Read the model definition and answer for the solid it produces. Units are mm, in the model's axes. A direction names the side the tool comes from. Round coordinates to 2 decimals unless told otherwise and drop trailing zeros. Loops run counter-clockwise (first coordinate to the right, second up) from the corner with the lowest first, then second, coordinate; pieces in that order, holes last. Notation, with made-up numbers: (72.5, 43.25) - (83.5, 43.25) arc R14 ccw to (83.5, 61.25) - close; hole circle Ø7 at (86.5, 56). An arc over 180 degrees is marked (long way). Answer as CSV lines item,"result".
```python
from build123d import *

# Parameters (mm, degrees)
BOSS_EXTRUDE1_DEPTH = 42
CUT_EXTRUDE1_REACH  = 70.337
SKETCH2_W           = 19
SKETCH2_H           = 33
SKETCH3_R           = 2.25
BOSS_EXTRUDE2_DEPTH = 8.75
FILLET1_R           = 0.5


with BuildPart() as part:
    # Sketch1 → Boss-Extrude1 (new body)
    with BuildSketch(Plane.XY):
        Polygon((19.580645161, 0), (19.580645161, 6.5), (4.580645161, 6.5), (4.580645161, 0), (-8.419354839, 0), (-8.419354839, 3), (-8.419354839, 35), (1.580645161, 35), (22.580645161, 35), (22.580645161, 3), (32.580645161, 3), (32.580645161, 0), align=None)
    extrude(amount=BOSS_EXTRUDE1_DEPTH)

    # Cut-Extrude1: up to this face of the body (flat: up to its plane)
    cut_extrude1_end = Plane(part.part.faces().sort_by_distance((4.580645161, 3.25, 21))[0])
    # Sketch2 → Cut-Extrude1 (cut, up to the picked face)
    with BuildSketch(Plane(origin=(32.580645161, 0, 0), x_dir=(0, 0, -1), z_dir=(1, 0, 0)), mode=Mode.PRIVATE) as cut_extrude1_sk1:
        with Locations((-21, 16.5)):
            Rectangle(SKETCH2_W, SKETCH2_H)
    cut_extrude1_tool1 = split(extrude(cut_extrude1_sk1.sketch, amount=-CUT_EXTRUDE1_REACH, mode=Mode.PRIVATE), bisect_by=cut_extrude1_end, keep=Keep.BOTH, mode=Mode.PRIVATE)
    add(cut_extrude1_tool1.solids().sort_by(Axis((32.580645, 16.5, 21), (-1, 0, 0)))[0], mode=Mode.SUBTRACT)

    # Sketch3 → Boss-Extrude2 (add)
    with BuildSketch(Plane(origin=(0, 35, 0), x_dir=(1, 0, 0), z_dir=(0, 1, 0))):
        with Locations(Location((-2.051707365, -21, 0), (0, 0, 90))):
            Circle(SKETCH3_R)
    extrude(amount=BOSS_EXTRUDE2_DEPTH)

    # Fillet1
    fillet1_edges = [part.edges().sort_by_distance(p)[0] for p in [
        (-2.051707365, 35, 23.25),
    ]]
    fillet(fillet1_edges, radius=FILLET1_R)


solid = part.part
```
1) A cutting plane is placed at C-C, the plane y = 23.5. Determine the outline of the cut face in (x, z), plus the area to 3 significant figures.
Entries:
outline,"(-8.42, 0) - (22.58, 0) - (22.58, 11.5) - (4.58, 11.5) - (4.58, 30.5) - (22.58, 30.5) - (22.58, 42) - (-8.42, 42) - close"
area,"960 mm^2"
2) Find the intervals of material crossed by line 1 (Z direction, x = 10, y = 17); line 2 (Y direction, x = 28.5, z = 5.5); line 3 (Y direction, x = 18.5, z = 18), in increasing order.
Entries:
line 1,"z = 0 to 11.5, 30.5 to 42"
line 2,"y = 0 to 3"
line 3,"y = 33 to 35"
3) Each of these flat-tipped pins is pushed along its axis until it touches: P1, Ø12.5, axis at x = 13, z = 7.5, coming from the -Y side; P2, Ø11, axis at x = 26, z = 39, coming from the +Y side; P3, Ø6, axis at y = 32.5, z = 12.5, coming from the +X side. Where does it stop, or does it pass through?
Entries:
P1,"stops at y = 6.5"
P2,"stops at y = 35"
P3,"stops at x = 22.58"
4) A cutting plane is placed at A-A, the plane z = 21. Determine the outline of the cut face in (x, y), plus the area to 3 significant figures.
Entries:
outline,"(-8.42, 0) - (4.58, 0) - (4.58, 33) - (22.58, 33) - (22.58, 35) - (0.7, 35) arc R0.5 cw to (0.2, 35.5) - (0.2, 43.75) - (-4.3, 43.75) - (-4.3, 35.5) arc R0.5 cw to (-4.8, 35) - (-8.42, 35) - close"
area,"530 mm^2"
5) The mould has two halves that part along X. Classify faces 6 (the face through (-8.419, 18, 21)), 7 (the face through (26, 0, 36)), 8 (the face through (32.581, 2, 6)), 9 (the face through (19.581, 3, 36)): pulls with the +X half, pulls with the -X half, needs draft (parallel to the pull), parting line crosses it, or undercut.
Entries:
face 6,"pulls with the -X half"
face 7,"needs draft"
face 8,"pulls with the +X half"
face 9,"undercut"
6) A cutting plane is placed at D-D, the plane z = 13. Determine the outline of the cut face in (x, y), plus the area to 3 significant figures.
Entries:
outline,"(-8.42, 0) - (4.58, 0) - (4.58, 33) - (22.58, 33) - (22.58, 35) - (-8.42, 35) - close"
area,"491 mm^2"
7) A tool of negligible diameter and unlimited length cuts with its end or side. For faces 1 (the face through (16, 16, 11.5)), 2 (the face through (4.581, 13, 21)), 3 (the face through (-2.728, 39.567, 18.854)), 4 (the face through (19.581, 3, 6)), 5 (the face through (28, 3, 36)), from which of +Z, -Z, +X, -X, +Y, -Y can it reach the whole face along a straight path? Write none if from no direction.
Entries:
face 1,"+X, -Y"
face 2,"-Y"
face 3,"+Y"
face 4,"+Z, -Z, -Y"
face 5,"+Z, -Z, +X, +Y"
8) A cutting plane is placed at B-B, the plane x = 7. Determine the outline of the cut face in (y, z), plus the area to 4 significant figures.
Entries:
outline,"(6.5, 0) - (35, 0) - (35, 42) - (6.5, 42) - (6.5, 30.5) - (33, 30.5) - (33, 11.5) - (6.5, 11.5) - close"
area,"693.5 mm^2"
